Autodesk Inventor part; units mm, degrees
ref_plane "РабПлоскость1" through (0, 0, 39.2) normal (0, 0, 1) x (1, 0, 0)
ref_plane "YZ Plane" through (0, 0, 0) normal (1, 0, 0) x (0, 1, 0)
ref_plane "XZ Plane" through (0, 0, 0) normal (0, 1, 0) x (-1, 0, 0)
ref_plane "РабПлоскость1" through (0, 0, 39.2) normal (0, 0, 1) x (1, 0, 0)
sketch "Эскиз1" plane through (0, 0, 39.2) normal (0, 0, 1) x (1, 0, 0)
  line L0 (27.5, -32.5) -> (-27.5, -32.5)
  line L1 (-32.5, -27.5) -> (-32.5, 27.5)
  line L2 (-27.5, 32.5) -> (27.5, 32.5)
  line L3 (32.5, 27.5) -> (32.5, -27.5)
  line L4 (32.5, -32.5) -> (-32.5, 32.5) construction
  line L5 (-32.5, -32.5) -> (32.5, 32.5) construction
  circle A0 centre (-15.35, 15.35) radius 1.75 construction
  circle A1 centre (15.35, 15.35) radius 1.75 construction
  arc A2 (14.0855, -15.35) -> (14.4559, -14.4559) centre (15.35, -15.35) ccw construction
  arc A3 (-16.6145, -15.35) -> (-16.2441, -14.4559) centre (-15.35, -15.35) ccw construction
  line L6 (-27.5, 32.5) -> (-32.5, 27.5)
  line L7 (-32.5, -27.5) -> (-27.5, -32.5)
  line L8 (27.5, -32.5) -> (32.5, -27.5)
  line L9 (27.5, 32.5) -> (32.5, 27.5)
  circle A4 centre (0, 0) radius 10.7 construction
  circle A5 centre (0, 0) radius 8.46 construction
  circle A6 centre (0, 0) radius 11.5
  dimension "d0" = 65
  dimension "d1" = 5
  dimension "d2" = 5
  dimension "d3" = 5
  dimension "d4" = 5
  dimension "d5" = 5
  dimension "d6" = 5
  dimension "d7" = 5
  dimension "d8" = 5
  dimension "d9" = 23
extrude "Выдавливание1" add sketch "Эскиз1" along normal blind 4
sketch "Эскиз2" plane through (0, 0, 43.2) normal (0, 0, 1) x (1, 0, 0)
  line L0 (15.35, -15.35) -> (-15.35, -15.35) construction
  line L1 (-15.35, -15.35) -> (-15.35, 15.35) construction
  line L2 (-15.35, 15.35) -> (15.35, 15.35) construction
  line L3 (15.35, 15.35) -> (15.35, -15.35) construction
  line L4 (15.35, -15.35) -> (-15.35, 15.35) construction
  line L5 (-15.35, -15.35) -> (15.35, 15.35) construction
  point P0 (0, 0)
  dimension "d12" = 30.7
hole "Отверстие1" at (-15.35, 15.35, 43.2) at (15.35, 15.35, 43.2) at (15.35, -15.35, 43.2) at (-15.35, -15.35, 43.2) direction (0, 0, -1) diameter 3.4 end through all countersink diameter 6.6 countersink angle 90
sketch "Эскиз3" plane through (0, 0, 43.2) normal (0, 0, 1) x (1, 0, 0)
  line L0 (26.4645, -26.4645) -> (-26.4645, -26.4645) construction
  line L1 (-26.4645, -26.4645) -> (-26.4645, 26.4645) construction
  line L2 (-26.4645, 26.4645) -> (26.4645, 26.4645) construction
  line L3 (26.4645, 26.4645) -> (26.4645, -26.4645) construction
  line L4 (26.4645, -26.4645) -> (-26.4645, 26.4645) construction
  line L5 (-26.4645, -26.4645) -> (26.4645, 26.4645) construction
  line L6 (-27.5, 32.5) -> (-32.5, 27.5) construction
  point P0 (0, 0)
  point P1 (-30, 30)
  dimension "d31" = 5
hole "Отверстие2" at (-26.4645, 26.4645, 43.2) at (26.4645, 26.4645, 43.2) at (26.4645, -26.4645, 43.2) at (-26.4645, -26.4645, 43.2) direction (0, 0, -1) diameter 3.9 end through all
sketch "Эскиз4" plane through (0, 0, 43.2) normal (0, 0, 1) x (1, 0, 0)
  circle A0 centre (0, 0) radius 12.5
  circle A1 centre (0, 0) radius 11.5
  dimension "d28" = 1
extrude "Выдавливание2" add sketch "Эскиз4" along normal blind 1
equation "\"d2\" = d1"
equation "\"d3\" = d1"
equation "\"d4\" = d3"
equation "\"d5\" = d1"
equation "\"d6\" = d5"
equation "\"d7\" = d1"
equation "\"d8\" = d7"
properties part number "Основание_нижнее" material "По умолчанию1"
Verification items for the finished model (mm, model axes). A direction names the side the tool comes from. Give positions to 0.01 mm unless a question says otherwise; leave off trailing zeros. Write each loop counter-clockwise with the first axis right and the second up, starting at its lowest first coordinate (ties: lowest second). Pieces come first, ordered by that corner, then holes. Notation, with made-up numbers: M 0,44 L 47,44 A8 ccw 47,53 Z; hole C 24.25,72 d1. An arc over 180 degrees is marked long. Put each result on its own line as item: value. Start each with the question number.
1. Scan lines: line 1 along X through (y, z) = (15.35, 40.95); line 2 along X through (y, z) = (-26.5, 42.7); line 3 along Y through (x, z) = (-15.5, 40.4). Record each from-to range of solid material in increasing order. Write a range as [from, to].
2. Section check C-C (x = 15.35). Record the cut outline in (y, z).
3. Go/stop test with flat-tipped pins: pin 1 Ø2 at (x, y) = (15.35, -15.35) entering from +Z; pin 2 Ø5 at (x, y) = (26.46, 26.46) entering from +Z; pin 3 Ø4 at (x, y) = (15.35, 15.35) entering from -Z. Record where each tip stops, or that it passes through.
4. Set-up check for faces 1 (the face through (27.651, -24.917, 41.172)), 2 (the face through (-15, 0, 43.2)): record each of +Z, -Z, +X, -X, +Y, -Y from which the full face is reachable in a straight line by a thin tool's end or side.
5. Section check A-A (x = 0). Record the cut outline in (y, z).
6. Draft check along X on faces 3 (the face through (-30, -30, 41)), 4 (the face through (30, -30, 41)), 5 (the face through (-25.278, 28.012, 41.172)). Enter one of: +X half, -X half, draft (parallel to the pull), parting line (faces both ways), or undercut.
Answer list:
1. line 1: [-32.5, -17.05], [-13.65, 13.65], [17.05, 32.5]
1. line 2: [-32.5, -28.41], [-24.51, 24.51], [28.41, 32.5]
1. line 3: [-32.5, -17.04], [-13.66, 13.66], [17.04, 32.5]
2. outline: M -32.5,39.2 L -17.05,39.2 L -17.05,41.6 L -18.65,43.2 L -32.5,43.2 Z; M -13.65,39.2 L 13.65,39.2 L 13.65,41.6 L 12.05,43.2 L -12.05,43.2 L -13.65,41.6 Z; M 17.05,39.2 L 32.5,39.2 L 32.5,43.2 L 18.65,43.2 L 17.05,41.6 Z
3. pin 1: through
3. pin 2: z = 43.2
3. pin 3: z = 39.2
4. face 1: +Z, -Z
4. face 2: +Z
5. outline: M -32.5,39.2 L -11.5,39.2 L -11.5,44.2 L -12.5,44.2 L -12.5,43.2 L -32.5,43.2 Z; M 11.5,39.2 L 32.5,39.2 L 32.5,43.2 L 12.5,43.2 L 12.5,44.2 L 11.5,44.2 Z
6. face 3: -X half
6. face 4: +X half
6. face 5: undercut
